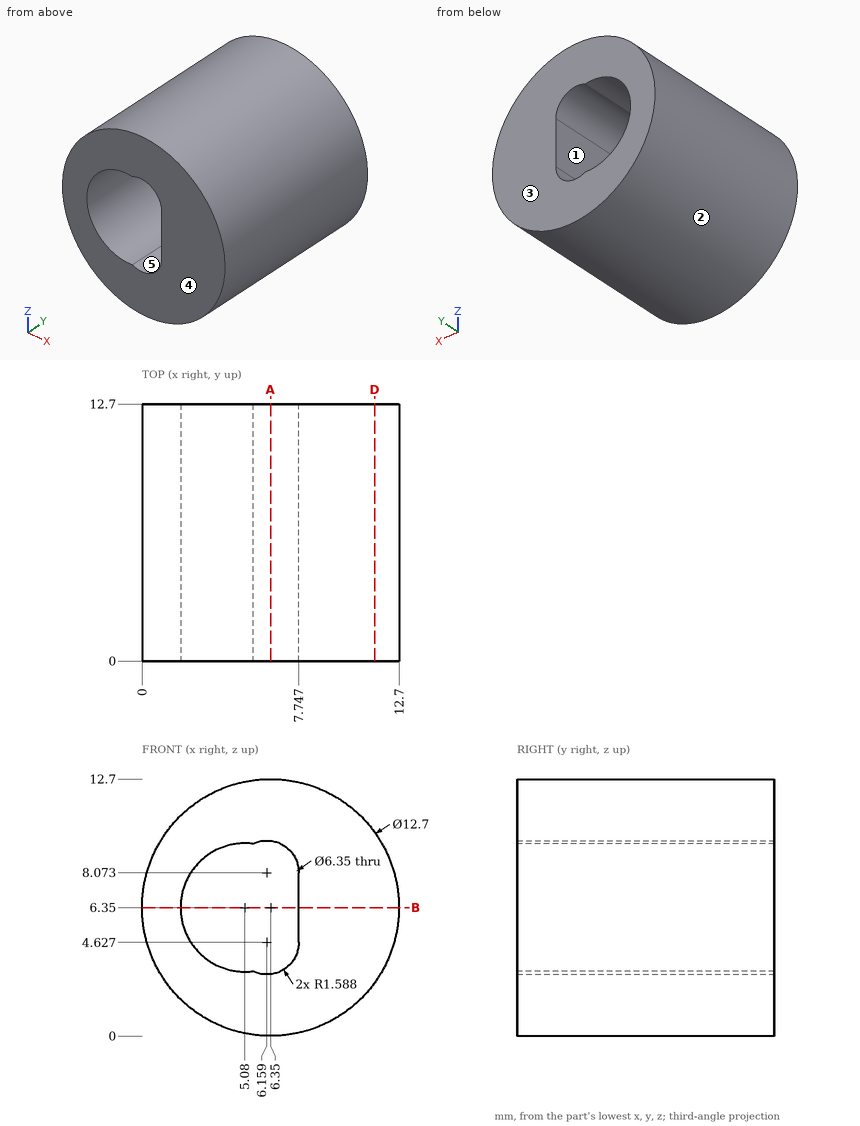
Can you work these out from the drawing? Everything is in mm from the part's minimum corner. A direction names the side the tool comes from. Give positions to 0.01 mm unless a question says otherwise; leave off trailing zeros. Loops run counter-clockwise (first coordinate to the right, second up) from the corner with the lowest first, then second, coordinate; pieces in that order, holes last. Notation, with made-up numbers: (74.25, 3) -> (117.25, 3) arc R18 ccw to (117.25, 8) -> close; hole circle Ø2 at (70.5, 2.25). An arc over 180 degrees is marked (long way). Return JSON: item names as keys, results as strings.
Q1. On a 3-axis mill with a long thin cutter (end or side, diameter ignored), from which of +Z, -Z, +X, -X, +Y, -Y can I reach the whole of each face in a straight line? I mean the marked faces 4 and 5. Say none if no direction works.
Checks:
{"face 4": "+Z, -Z, +X, -X, -Y", "face 5": "+Y, -Y"}
Q2. I want a section at A-A, the plane x = 6.35. List the corners of the cut face in (y, z) for me.
Checks:
{"outline": "(0, 0) -> (12.7, 0) -> (12.7, 3.05) -> (0, 3.05) -> close; (0, 9.65) -> (12.7, 9.65) -> (12.7, 12.7) -> (0, 12.7) -> close"}
Q3. I want a section at B-B, the plane z = 6.35. List the corners of the cut face in (x, y) for me (1 decimal).
Checks:
{"outline": "(0, 0) -> (1.9, 0) -> (1.9, 12.7) -> (0, 12.7) -> close; (7.7, 0) -> (12.7, 0) -> (12.7, 12.7) -> (7.7, 12.7) -> close"}
Q4. I need wall thicknesses on probe 1 along X at (y, z) = (6.25, 6.35) (1 decimal); probe 2 along X at (y, z) = (2.5, 8.5) (1 decimal); probe 3 along Z at (x, y) = (5.08, 4.25) (1 decimal). Which ranges of each line are inside material? Lowest first, please.
Checks:
{"probe 1": "x = 0 to 1.9, 7.7 to 12.7", "probe 2": "x = 0.4 to 2.7, 7.7 to 12.3", "probe 3": "z = 0.1 to 3.2, 9.5 to 12.6"}
Q5. We'd pull the mould along Z, two halves only. Please class the marked faces 1, 2 and 3: released by +Z, released by -Z, zero draft, split by the parting line, or undercut.
Checks:
{"face 1": "undercut", "face 2": "split by the parting line", "face 3": "zero draft"}
Q6. I want a section at D-D, the plane x = 11.5. List the corners of the cut face in (y, z) for me (1 decimal).
Checks:
{"outline": "(0, 2.6) -> (12.7, 2.6) -> (12.7, 10.1) -> (0, 10.1) -> close"}
Q7. For pin 1 Ø5 at (x, y) = (10.5, 8) entering from -Z; pin 2 Ø3 at (y, z) = (3.5, 11.5) entering from -X (1 decimal); pin 3 Ø2 at (x, y) = (3, 5.5) entering from +Z, each with a flat end and sliding along its axis, tell me the tip position at first contact or that it passes through.
Checks:
{"pin 1": "stops at z = 0.22", "pin 2": "stops at x = 1.2", "pin 3": "stops at z = 12.25"}
